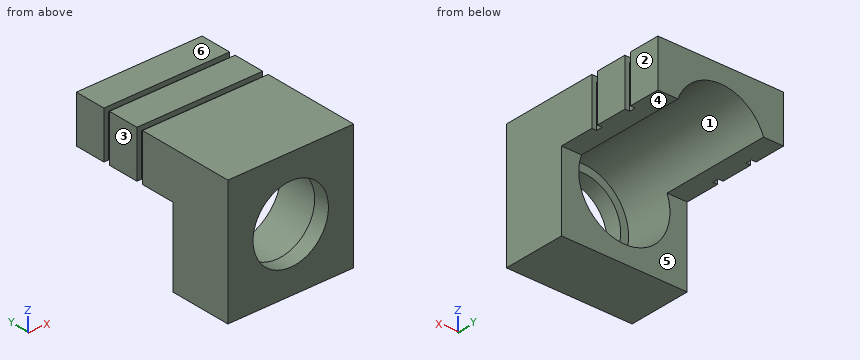
from build123d import *

# Parameters (mm, degrees)
BOSS_EXTRUDE2_DEPTH = 80
SKETCH5_R           = 29
CUT_EXTRUDE1_DEPTH  = 100
SKETCH6_R           = 24
CUT_EXTRUDE2_DEPTH  = 111
SKETCH7_W           = 30
SKETCH7_H           = 4
CUT_EXTRUDE3_DEPTH  = 3
SKETCH8_W           = 30
SKETCH8_H           = 4
CUT_EXTRUDE4_DEPTH  = 3
SKETCH9_W           = 74
SKETCH9_H           = 4
CUT_EXTRUDE5_DEPTH  = 3


with BuildPart() as part:
    # Sketch4 → Boss-Extrude2 (new body)
    with BuildSketch(Plane(origin=(0, 0, 0), x_dir=(0, 0, -1), z_dir=(1, 0, 0))):
        Polygon((0, 0), (80, 0), (80, 40), (30, 40), (30, 110), (0, 110), align=None)
    extrude(amount=BOSS_EXTRUDE2_DEPTH)

    # Sketch5 → Cut-Extrude1 (cut)
    with BuildSketch(Plane(origin=(0, 110, 0), x_dir=(1, 0, 0), z_dir=(0, 1, 0))):
        with Locations((40, 40)):
            Circle(SKETCH5_R)
    extrude(amount=-CUT_EXTRUDE1_DEPTH, mode=Mode.SUBTRACT)

    # Sketch6 → Cut-Extrude2 (cut, through all)
    with BuildSketch(Plane.XZ):
        with Locations((40, -40)):
            Circle(SKETCH6_R)
    extrude(amount=-CUT_EXTRUDE2_DEPTH, mode=Mode.SUBTRACT)

    # Sketch7 → Cut-Extrude3 (cut)
    with BuildSketch(Plane(origin=(80, 0, 0), x_dir=(0, 0, -1), z_dir=(1, 0, 0))):
        with Locations((15, 88)):
            Rectangle(SKETCH7_W, SKETCH7_H)
        with Locations((15, 64)):
            Rectangle(SKETCH7_W, SKETCH7_H)
    extrude(amount=-CUT_EXTRUDE3_DEPTH, mode=Mode.SUBTRACT)

    # Sketch8 → Cut-Extrude4 (cut)
    with BuildSketch(Plane.ZY):
        with Locations((-15, 88)):
            Rectangle(SKETCH8_W, SKETCH8_H)
        with Locations((-15, 64)):
            Rectangle(SKETCH8_W, SKETCH8_H)
    extrude(amount=-CUT_EXTRUDE4_DEPTH, mode=Mode.SUBTRACT)

    # Sketch9 → Cut-Extrude5 (cut)
    with BuildSketch(Plane.XY):
        with Locations((40, 88)):
            Rectangle(SKETCH9_W, SKETCH9_H)
        with Locations((40, 64)):
            Rectangle(SKETCH9_W, SKETCH9_H)
    extrude(amount=-CUT_EXTRUDE5_DEPTH, mode=Mode.SUBTRACT)


solid = part.part
Verification items for the finished model (mm, model axes). Face numbers are marked on the shaded views. A direction names the side the tool comes from. Coordinates: 2 decimals unless noted, no trailing zeros. Order: outer loops, then holes, each group sorted by start corner. A loop starts at its lowest first (then second) coordinate and runs counter-clockwise, first axis right, second up. Notation, with made-up numbers: (78, -0.5) -> (105, -0.5) arc R20 ccw to (105, 35.5) -> close; hole circle Ø11 at (9.5, 88.25). An arc over 180 degrees is marked (long way). Use CSV: the item, a comma, the result in double quotes. Start each with the question number.
Q1. Section check D-D, the plane y = 91.5. Record the cut outline in (x, z).
Q2. Section check B-B, the plane z = -40. Record the cut outline in (x, y).
Q3. Draft check along X on the marked faces 1, 2, 3 and 4. Enter one of: +X half, -X half, draft (parallel to the pull), parting line (faces both ways), or undercut.
Q4. Thickness scan on line 1 along X through (y, z) = (39.5, -40); line 2 along Z through (x, y) = (40, 33.5); line 3 along Y through (x, z) = (75.5, -41). Record the ranges inside material, lowest first.
Q5. Depth check by flat-ended pin: P1, Ø2, axis at y = 64, z = -11.5, coming from the +X side; P2, Ø10, axis at x = 8.5, y = 76.5, coming from the -Z side; P3, Ø1.2, axis at y = 87, z = -16, coming from the -X side. Enter the tip coordinate at first touch or a pass-through.
Q6. Section check C-C, the plane y = 37. Record the cut outline in (x, z), and give its area (3 significant figures).
Q7. Tool access check on the marked faces 5 and 6. Record the directions out of +Z, -Z, +X, -X, +Y, -Y that give a thin tool (end or side, any length) a straight path to the whole face; none if there is none.
Q8. Section check A-A, the plane x = 40. Record the cut outline in (y, z), and give its area (3 significant figures).
Returned:
1,outline,"(0, -30) -> (12.78, -30) arc R29 cw to (67.22, -30) -> (80, -30) -> (80, 0) -> (0, 0) -> close"
2,outline,"(0, 0) -> (16, 0) -> (16, 10) -> (11, 10) -> (11, 40) -> (0, 40) -> close; (64, 0) -> (80, 0) -> (80, 40) -> (69, 40) -> (69, 10) -> (64, 10) -> close"
3,face 1,"undercut"
3,face 2,"+X half"
3,face 3,"-X half"
3,face 4,"draft"
4,line 1,"x = 0 to 11, 69 to 80"
4,line 2,"z = -80 to -69, -11 to 0"
4,line 3,"y = 0 to 40"
5,P1,"stops at x = 77"
5,P2,"stops at z = -30"
5,P3,"stops at x = 3"
6,outline,"(0, -80) -> (80, -80) -> (80, 0) -> (0, 0) -> close; hole circle Ø58 at (40, -40)"
6,area,"3,760 mm^2"
7,face 5,"-Z, +X, -X, +Y"
7,face 6,"+Z, +X, -X, +Y, -Y"
8,outline,"(0, -80) -> (40, -80) -> (40, -69) -> (10, -69) -> (10, -64) -> (0, -64) -> close; (0, -16) -> (10, -16) -> (10, -11) -> (110, -11) -> (110, 0) -> (90, 0) -> (90, -3) -> (86, -3) -> (86, 0) -> (66, 0) -> (66, -3) -> (62, -3) -> (62, 0) -> (0, 0) -> close"
8,area,"1,730 mm^2"
